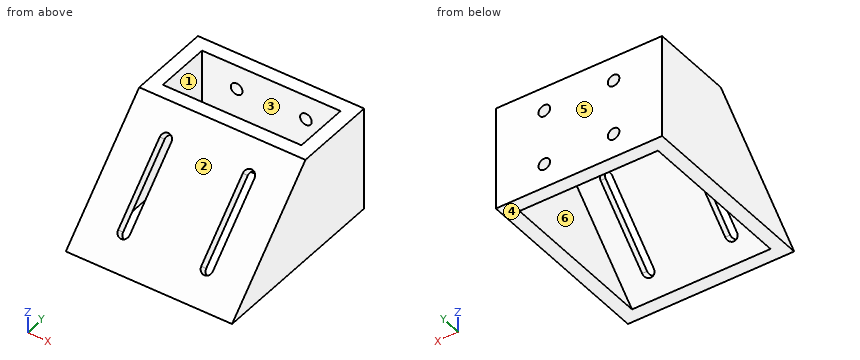
from build123d import *

# Parameters (mm, degrees)
EXTRUDE_1_DEPTH     = 5
EXTRUDE_3_DEPTH     = 50
CUT_EXTRUDE_2_DEPTH = 50
EXTRUDE_4_DEPTH     = 5
SKETCH_6_W          = 60
SKETCH_6_H          = 37.476659403
EXTRUDE_5_DEPTH     = 5
SKETCH_7_R          = 2.1
CUT_EXTRUDE_3_DEPTH = 5


with BuildPart() as part:
    # 草图2 → 凸台-拉伸1 (new body)
    with BuildSketch(Plane(origin=(0, 0, 0), x_dir=(0, 0, -1), z_dir=(1, 0, 0))):
        Polygon((0, 30), (0, 0), (37.476659403, -37.476659403), (37.476659403, 30), align=None)
    extrude(amount=EXTRUDE_1_DEPTH)

    # 草图4 → 凸台-拉伸3 (add)
    with BuildSketch(Plane(origin=(5, 0, 0), x_dir=(0, 0, -1), z_dir=(1, 0, 0))):
        Polygon((0, 0), (0, 5), (37.476659403, -32.476659403), (37.476659403, -37.476659403), align=None)
    extrude(amount=EXTRUDE_3_DEPTH)

    # 草图3 → 切除-拉伸2 (cut)
    with BuildSketch(Plane(origin=(0, 0, 0), x_dir=(1, 0, 0), z_dir=(0, -0.7071067811865489, 0.7071067811865462))):
        with BuildLine():
            ThreePointArc((17.1, -41), (15, -43.1), (12.9, -41))
            Line((12.9, -41), (12.9, -11))
            ThreePointArc((12.9, -11), (15, -8.9), (17.1, -11))
            Line((17.1, -11), (17.1, -41))
        make_face()
        with BuildLine():
            Line((42.9, -11), (42.9, -41))
            ThreePointArc((42.9, -41), (45, -43.1), (47.1, -41))
            Line((47.1, -41), (47.1, -11))
            ThreePointArc((47.1, -11), (45, -8.9), (42.9, -11))
        make_face()
    extrude(amount=-CUT_EXTRUDE_2_DEPTH, mode=Mode.SUBTRACT)

    # 草图5 → 凸台-拉伸4 (add)
    with BuildSketch(Plane(origin=(55, 0, 0), x_dir=(0, 0, -1), z_dir=(1, 0, 0))):
        Polygon((0, 30), (0, 0), (37.476659403, -37.476659403), (37.476659403, 30), align=None)
    extrude(amount=EXTRUDE_4_DEPTH)

    # 草图6 → 凸台-拉伸5 (add)
    with BuildSketch(Plane(origin=(0, 30, 0), x_dir=(1, 0, 0), z_dir=(0, 1, 0))):
        with Locations((30, 18.738329701)):
            Rectangle(SKETCH_6_W, SKETCH_6_H)
    extrude(amount=-EXTRUDE_5_DEPTH)

    # 草图7 → 切除-拉伸3 (cut)
    with BuildSketch(Plane(origin=(0, 30, 0), x_dir=(1, 0, 0), z_dir=(0, 1, 0))):
        with Locations(Location((42.5, 28.738329701, 0), (0, 0, 270))):
            Circle(SKETCH_7_R)
        with Locations(Location((17.5, 28.738329701, 0), (0, 0, 90))):
            Circle(SKETCH_7_R)
        with Locations(Location((42.5, 8.738329701, 0), (0, 0, 90))):
            Circle(SKETCH_7_R)
        with Locations(Location((17.5, 8.738329701, 0), (0, 0, 270))):
            Circle(SKETCH_7_R)
    extrude(amount=-CUT_EXTRUDE_3_DEPTH, mode=Mode.SUBTRACT)


solid = part.part
Could you check a few things on this model? Use its own coordinates, in mm. Face numbers are marked on the shaded views. A direction names the side the tool comes from. Round coordinates to 2 decimals unless told otherwise and drop trailing zeros. Write each loop counter-clockwise with the first axis right and the second up, starting at its lowest first coordinate (ties: lowest second). Pieces come first, ordered by that corner, then holes. Notation, with made-up numbers: (78.5, 41) - (105.5, 41) arc R10 cw to (105.5, 50) - close; hole circle Ø11 at (67, 71.5). An arc over 180 degrees is marked (long way). Put each result on its own line as item: value. Start each with the question number.
(1) I need wall thicknesses on probe 1 along X at (y, z) = (17, -12.5); probe 2 along Z at (x, y) = (42, 28); probe 3 along Y at (x, z) = (16, -26). Which ranges of each line are inside material? Lowest first, please.
(2) Will these pins go through, and if not, where does the flat tip stop? pin 1 (3.5 mm diameter, centred on x = 17.5, z = -8.74, fed in from -Y); pin 2 (18.5 mm diameter, centred on x = 37, z = -15.5, fed in from -Y); pin 3 (8 mm diameter, centred on x = 19.5, z = -22.5, fed in from -Y).
(3) I want a section at A-A, the plane x = 27.5. Please give me the cut outline in (y, z), plus the area to 3 significant figures.
(4) I want a section at C-C, the plane z = -4. Please give me the cut outline in (x, y).
(5) Thinking about a two-plate mould opening in Y: for the marked faces 4, 5 and 6, which applies, released by +Y, released by -Y, zero draft, split by the parting line, or undercut?
(6) For the marked faces 1, 2 and 3, which set-ups out of +Z, -Z, +X, -X, +Y, -Y let a thin tool reach every point of the face, with its end or its side?
(7) I want a section at B-B, the plane y = -23.5. Please give me the cut outline in (x, z).
Here are the results:
1. probe 1: x = 0 to 5, 55 to 60
1. probe 2: z = -37.48 to -30.78, -26.7 to -10.78, -6.7 to 0
1. probe 3: y = 25 to 30
2. pin 1: stops at y = -10.49
2. pin 2: stops at y = -24.75
2. pin 3: stops at y = -26.5
3. outline: (-37.48, -37.48) - (-32.48, -37.48) - (5, 0) - (0, 0) - close; (25, -37.48) - (30, -37.48) - (30, 0) - (25, 0) - close
3. area: 375 mm^2
4. outline: (0, -4) - (60, -4) - (60, 30) - (0, 30) - close; hole (5, 1) - (55, 1) - (55, 25) - (5, 25) - close
5. face 4: zero draft
5. face 5: released by +Y
5. face 6: undercut
6. face 1: -Z
6. face 2: +Z, +X, -X, -Y
6. face 3: +Z, -Z
7. outline: (0, -37.48) - (5, -37.48) - (5, -28.5) - (12.9, -28.5) - (12.9, -23.5) - (0, -23.5) - close; (17.1, -28.5) - (42.9, -28.5) - (42.9, -23.5) - (17.1, -23.5) - close; (47.1, -28.5) - (55, -28.5) - (55, -37.48) - (60, -37.48) - (60, -23.5) - (47.1, -23.5) - close
